Source: three-view drawing plus pictorial views. Frame: mm from the lowest corner of the part. Give positions to 0.01 mm unless a question says otherwise; leave off trailing zeros. Order: outer loops, then holes, each group sorted by start corner. A loop starts at its lowest first (then second) coordinate and runs counter-clockwise, first axis right, second up. Notation, with made-up numbers: (3.25, 13.5) - (12.25, 13.5) arc R22 cw to (12.25, 47.5) - close; hole circle Ø11 at (20.5, 39). An arc over 180 degrees is marked (long way). Answer in a Markdown table with one row per item. Add a question column.
1. Contact query for flat-ended pins moving along their axis: pin 1 (1 mm diameter, centred on y = 9, z = 3, fed in from -X); pin 2 (2 mm diameter, centred on x = 27.5, z = 2.5, fed in from -Y). Output: stop coordinate, or through.
2. Ray query, line 1 (Y direction, x = 37, z = 1.2); line 2 (X direction, y = 33.5, z = 2.1); line 3 (Y direction, x = 8.5, z = 1.5). Return the intervals inside material, ascending. Write a range as [from, to].
3. Section query C-C on z = 4.3. Return loops of the section in (x, y), and give its area (3 significant figures).
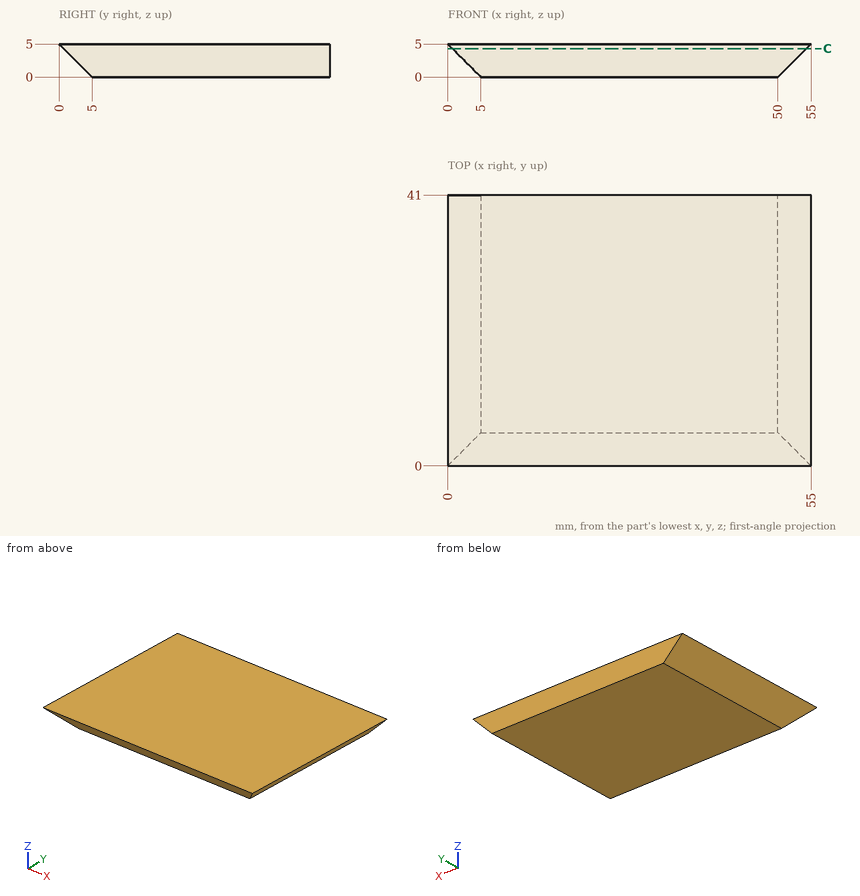
Answer:
| question | item | result |
|---|---|---|
| 1 | pin 1 | stops at x = 1.5 |
| 1 | pin 2 | stops at y = 1.5 |
| 2 | line 1 | y = [3.8, 41] |
| 2 | line 2 | x = [2.9, 52.1] |
| 2 | line 3 | y = [3.5, 41] |
| 3 | outline | (0.7, 0.7) - (54.3, 0.7) - (54.3, 41) - (0.7, 41) - close |
| 3 | area | 2,160 mm² |
